Design review of the part built by this model. Coordinates are the model's own, in mm. Give positions to 0.01 mm unless a question says otherwise; leave off trailing zeros. Loops run counter-clockwise (first coordinate to the right, second up) from the corner with the lowest first, then second, coordinate; pieces in that order, holes last. Notation, with made-up numbers: (-1.5, 20) - (57.5, 20) arc R10 ccw to (57.5, 28) - close; hole circle Ø1 at (64, 71.5). An arc over 180 degrees is marked (long way). One line per item, written item: value. Start each with the question number.
```python
from build123d import *

# Parameters (mm, degrees)
F0_W     = 52.832
F0_H     = 103.886
F1_DEPTH = 0.79375
F2_W     = 7.6454
F2_H     = 17.1704
F2_H_2   = 7.5184
F2_W_2   = 2.405321
F2_H_3   = 37.719
F2_W_3   = 2.413
F2_H_4   = 28.067
F2_R     = 1.5875
F3_DEPTH = 1.6002


with BuildPart() as f1:
    # F0 (on Top) → F1 (new body, symmetric)
    with BuildSketch(Plane.XY):
        Rectangle(F0_W, F0_H)
    extrude(amount=F1_DEPTH, both=True)

    # F2 (on face) → F3 (cut)
    with BuildSketch(Plane.XY.offset(0.79375)):
        with Locations((-22.5933, 43.3578)):
            Rectangle(F2_W, F2_H)
        with Locations((22.5933, 48.1838)):
            Rectangle(F2_W, F2_H_2)
        Polygon((-26.416, -44.4246), (-26.416, -51.943), (-18.7706, -51.943), (-18.7706, -44.4246), (-24.010679, -44.4246), align=None)
        with Locations((-25.21334, -25.5651)):
            Rectangle(F2_W_2, F2_H_3)
        Polygon((18.7706, -51.943), (26.416, -51.943), (26.416, -34.7726), (24.003, -34.7726), (18.7706, -34.7726), align=None)
        with Locations((25.2095, -20.7391)):
            Rectangle(F2_W_3, F2_H_4)
        with Locations((-15.567212, 48.84192)):
            Circle(F2_R)
        with Locations((15.567212, 48.84192)):
            Circle(F2_R)
        with Locations((-15.567212, -48.84192)):
            Circle(F2_R)
        with Locations((15.567212, -48.84192)):
            Circle(F2_R)
    extrude(amount=-F3_DEPTH, mode=Mode.SUBTRACT)


solid = f1.part
```
(1) Draft analysis for pull direction Y (two halves, no side actions). For faces 1 (the cylindrical face through (14.397, -47.769, 0.011)), 2 (the flat face through (0, 1, -0.794)), state which applies: pulls with the +Y half, pulls with the -Y half, needs draft (parallel to the pull), parting line crosses it, or undercut.
(2) For pin 1 Ø0.5 at (x, z) = (-21, -0.5) entering from -Y; pin 2 Ø0.5 at (x, z) = (22.5, 0.5) entering from -Y; pin 3 Ø0.5 at (y, z) = (-41.5, 0) entering from +X, all flat-tipped, find the tip position at first contact; note any pin that passes through.
(3) Take a section at A-A on z = -0.25. State the section outline as (x, y) points (1 decimal).
(4) Take a section at C-C on y = 42.5. State the section outline as (x, z) points.
(5) Take a section at B-B on x = -21. State the section outline as (y, z) points, and give its area (3 significant figures).
(6) To check wall thickness, follow L1, parallel to Y at x = 14.5, z = -0.4; L2, parallel to X at y = -43, z = -0.4; L3, parallel to Y at x = 16.5, z = -0.6. State the ranges of each line that lie inside material, in increasing order. Write a range as from..to.
Here are the results:
1. face 1: undercut
1. face 2: needs draft
2. pin 1: y = -44.42
2. pin 2: y = -34.77
2. pin 3: x = 18.77
3. outline: (-26.4, -6.7) - (-24, -6.7) - (-24, -44.4) - (-18.8, -44.4) - (-18.8, -51.9) - (18.8, -51.9) - (18.8, -34.8) - (24, -34.8) - (24, -6.7) - (26.4, -6.7) - (26.4, 44.4) - (18.8, 44.4) - (18.8, 51.9) - (-18.8, 51.9) - (-18.8, 34.8) - (-26.4, 34.8) - close; hole circle Ø3.2 at (-15.6, -48.8); hole circle Ø3.2 at (-15.6, 48.8); hole circle Ø3.2 at (15.6, -48.8); hole circle Ø3.2 at (15.6, 48.8)
4. outline: (-18.77, -0.79) - (26.42, -0.79) - (26.42, 0.79) - (-18.77, 0.79) - close
5. outline: (-44.42, -0.79) - (34.77, -0.79) - (34.77, 0.79) - (-44.42, 0.79) - close
5. area: 126 mm²
6. L1: -51.94..-50.02, -47.67..47.67, 50.02..51.94
6. L2: -24.01..18.77
6. L3: -51.94..-50.13, -47.56..47.56, 50.13..51.94
